from build123d import *

# Parameters (mm, degrees)
F1_DEPTH = 9.525
F2_R     = 1.5875
F4_DEPTH = 6.35


with BuildPart() as f1:
    # F0 (on Right) → F1 (new body, symmetric)
    with BuildSketch(Plane.YZ):
        Polygon((0, 3.175), (0, 0), (26.542, 0), (26.542, 32.258), (0, 32.258), (0, 29.083), (23.367, 29.083), (23.367, 3.175), align=None)
    extrude(amount=F1_DEPTH, both=True)

    # F2
    f2_edges = [f1.edges().sort_by_distance(p)[0] for p in [
        (9.525, 0, 30.6705),
        (-9.525, 0, 30.6705),
        (-9.525, 0, 1.5875),
        (9.525, 0, 1.5875),
        (0, 26.542, 32.258),
        (0, 26.542, 0),
    ]]
    fillet(f2_edges, radius=F2_R)

    # F3 (on Right) → F4 (join, symmetric)
    with BuildSketch(Plane.YZ):
        with BuildLine():
            Line((13.404685, 16.92275), (5.467418, 3.175))
            Line((5.467418, 3.175), (11.817418, 3.175))
            Line((11.817418, 3.175), (10.475505, 5.499261))
            ThreePointArc((10.475505, 5.499261), (10.050135, 7.086761), (10.475505, 8.674261))
            Line((10.475505, 8.674261), (13.98575, 14.754185))
            ThreePointArc((13.98575, 14.754185), (16.312907, 16.539875), (13.404685, 16.92275))
        make_face()
    extrude(amount=F4_DEPTH, both=True)

    # F5 (on Right) → F6 (revolve)
    with BuildSketch(Plane.YZ):
        Polygon((8.642418, 0), (3.879918, 0), (3.879918, -43.4975), (8.642418, -48.26), align=None)
    revolve(axis=Axis((0, 8.642418, -24.13), (0, 0, 1)))


solid = f1.part
Build history of the part. All positions in model axes, mm. A direction names the side the tool comes from. Give positions to 0.01 mm unless a question says otherwise; leave off trailing zeros. Order: outer loops, then holes, each group sorted by start corner. A loop starts at its lowest first (then second) coordinate and runs counter-clockwise, first axis right, second up. Notation, with made-up numbers: M 72.5,22.25 L 111.5,22.25 A35 ccw 111.5,59.25 Z; hole C -7,25 d3. An arc over 180 degrees is marked long. Put each result on its own line as item: value.
Item 1: Probe line 1 (Z direction, x = -7.25, y = 7.25) (3 decimals); line 2 (Z direction, x = 0.5, y = 14.5) (3 decimals); line 3 (Z direction, x = 0.5, y = 14.25) (3 decimals). List the from-to ranges inside material, lowest first. Write a range as [from, to].
From the geometry:
line 1: z = [0, 3.175], [29.083, 32.258]
line 2: z = [0, 3.175], [14.566, 17.692], [29.083, 32.258]
line 3: z = [0, 3.175], [14.632, 17.626], [29.083, 32.258]
Item 2: Flat gauge pins, fed straight in: pin 1 Ø1.5 at (y, z) = (4.5, 6) entering from -X; pin 2 Ø1 at (x, y) = (0, 22) entering from -Z; pin 3 Ø6 at (x, z) = (3.5, 9) entering from -Y; pin 4 Ø4 at (x, z) = (-1, 15.5) entering from -Y. Where does each tip first touch, or does it go through?
From the geometry:
pin 1: passes through
pin 2: stops at z = 0
pin 3: stops at y = 7.1
pin 4: stops at y = 11.43
Item 3: Slice it at A-A, the plane y = 17.25. Write the cut outline in (x, z) (3 decimals).
From the geometry:
outline: M -9.525,0 L 9.525,0 L 9.525,3.175 L -9.525,3.175 Z; M -9.525,29.083 L 9.525,29.083 L 9.525,32.258 L -9.525,32.258 Z
Item 4: Slice it at B-B, the plane z = 24.5. Write the cut outline in (x, y) (3 decimals), plus the area to 3 significant figures.
From the geometry:
outline: M -9.525,23.367 L 9.525,23.367 L 9.525,26.542 L -9.525,26.542 Z
area: 60.5 mm2
Item 5: 3-axis set-ups, long thin cutter, end or side, ignore diameter. For faces 4 (the cylindrical face through (9.048, 0.453, 1.565)), 5 (the flat face through (0.089, 9.492, 10.145)), 6 (the flat face through (-6.35, 11, 10)), 7 (the cylindrical face through (0.09, 10.05, 7.06)), 8 (the cylindrical face through (-2.9, 12.42, -22.05)): which of +Z, -Z, +X, -X, +Y, -Y reach the whole face in a straight line?
From the geometry:
face 4: +Z, -Z, +X, -Y
face 5: +X, -X, -Y
face 6: -X, -Y
face 7: +X, -X
face 8: -Z
Item 6: Two-plate mould, pull along Y, no slides. Class faces 1 (the flat face through (0, 12, 29.083)), 2 (the flat face through (0.089, 11.156, 4.321)), 3 (the flat face through (0, 26.542, 16)): +Y half, -Y half, draft (parallel to the pull), parting line (faces both ways), or undercut.
From the geometry:
face 1: draft
face 2: undercut
face 3: +Y half
Item 7: Slice it at C-C, the plane z = -32. Write the cut outline in (x, y) (1 decimal).
From the geometry:
outline: C 0,8.6 d9.5
